Work out the finished part from the listing and answer in its coordinate system (mm). Give positions to 0.01 mm unless a question says otherwise; leave off trailing zeros. Loops run counter-clockwise (first coordinate to the right, second up) from the corner with the lowest first, then second, coordinate; pieces in that order, holes last. Notation, with made-up numbers: M -33.75,53.25 L 25.25,53.25 A19 ccw 25.25,80.25 Z; hole C -16.75,-24.5 d6. An arc over 180 degrees is marked long. Answer as a JSON object with one key per item and string values. Group by question number.
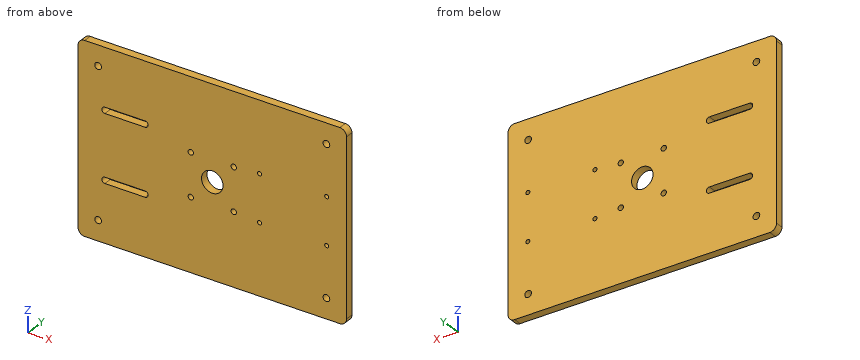
```python
from build123d import *

# Parameters (mm, degrees)
SKETCH2_W           = 200
SKETCH2_H           = 140
BOSS_EXTRUDE1_DEPTH = 6
FILLET1_R           = 5
SKETCH3_R           = 2.5
CUT_EXTRUDE1_DEPTH  = 123.21292894
SKETCH4_R           = 8
CUT_EXTRUDE2_DEPTH  = 123.21292894
SKETCH5_R           = 2
CUT_EXTRUDE3_DEPTH  = 123.21292894
CUT_EXTRUDE4_DEPTH  = 123.21292894
SKETCH7_R           = 1.5
CUT_EXTRUDE5_DEPTH  = 123.21292894


with BuildPart() as part:
    # Sketch2 → Boss-Extrude1 (new body)
    with BuildSketch(Plane(origin=(0, 0, 0), x_dir=(1, 0, 0), z_dir=(0, 1, 0))):
        Rectangle(SKETCH2_W, SKETCH2_H)
    extrude(amount=BOSS_EXTRUDE1_DEPTH)

    # Fillet1
    fillet1_edges = [part.edges().sort_by_distance(p)[0] for p in [
        (100, 3, 70),
        (-100, 3, 70),
        (-100, 3, -70),
        (100, 3, -70),
    ]]
    fillet(fillet1_edges, radius=FILLET1_R)

    # Sketch3 → Cut-Extrude1 (cut, through all)
    with BuildSketch(Plane(origin=(0, 6, 0), x_dir=(1, 0, 0), z_dir=(0, 1, 0))):
        with Locations(Location((-85, 55, 0), (0, 0, 270))):
            Circle(SKETCH3_R)
        with Locations(Location((-85, -55, 0), (0, 0, 90))):
            Circle(SKETCH3_R)
        with Locations(Location((85, -55, 0), (0, 0, 270))):
            Circle(SKETCH3_R)
        with Locations(Location((85, 55, 0), (0, 0, 90))):
            Circle(SKETCH3_R)
    extrude(amount=-CUT_EXTRUDE1_DEPTH, mode=Mode.SUBTRACT)

    # Sketch4 → Cut-Extrude2 (cut, through all)
    with BuildSketch(Plane(origin=(0, 6, 0), x_dir=(1, 0, 0), z_dir=(0, 1, 0))):
        with Locations(Location((0, 0, 0), (0, 0, 270))):
            Circle(SKETCH4_R)
    extrude(amount=-CUT_EXTRUDE2_DEPTH, mode=Mode.SUBTRACT)

    # Sketch5 → Cut-Extrude3 (cut, through all)
    with BuildSketch(Plane(origin=(0, 6, 0), x_dir=(1, 0, 0), z_dir=(0, 1, 0))):
        with Locations(Location((16, 16, 0), (0, 0, 270))):
            Circle(SKETCH5_R)
        with Locations(Location((16, -16, 0), (0, 0, 270))):
            Circle(SKETCH5_R)
        with Locations(Location((-16, -16, 0), (0, 0, 270))):
            Circle(SKETCH5_R)
        with Locations(Location((-16, 16, 0), (0, 0, 270))):
            Circle(SKETCH5_R)
    extrude(amount=-CUT_EXTRUDE3_DEPTH, mode=Mode.SUBTRACT)

    # Sketch6 → Cut-Extrude4 (cut, through all)
    with BuildSketch(Plane(origin=(0, 6, 0), x_dir=(1, 0, 0), z_dir=(0, 1, 0))):
        with BuildLine():
            Line((-80, 27.25), (-50, 27.25))
            ThreePointArc((-50, 27.25), (-47.75, 25), (-50, 22.75))
            Line((-50, 22.75), (-80, 22.75))
            ThreePointArc((-80, 22.75), (-82.25, 25), (-80, 27.25))
        make_face()
        with BuildLine():
            Line((-80, -22.75), (-50, -22.75))
            ThreePointArc((-50, -22.75), (-47.75, -25), (-50, -27.25))
            Line((-50, -27.25), (-80, -27.25))
            ThreePointArc((-80, -27.25), (-82.25, -25), (-80, -22.75))
        make_face()
    extrude(amount=-CUT_EXTRUDE4_DEPTH, mode=Mode.SUBTRACT)

    # Sketch7 → Cut-Extrude5 (cut, through all)
    with BuildSketch(Plane(origin=(0, 6, 0), x_dir=(1, 0, 0), z_dir=(0, 1, 0))):
        with Locations(Location((35.22226737, -17.5, 0), (0, 0, 270))):
            Circle(SKETCH7_R)
        with Locations(Location((35.22226737, 17.5, 0), (0, 0, 270))):
            Circle(SKETCH7_R)
        with Locations(Location((85.22226737, 17.5, 0), (0, 0, 270))):
            Circle(SKETCH7_R)
        with Locations(Location((85.22226737, -17.5, 0), (0, 0, 270))):
            Circle(SKETCH7_R)
    extrude(amount=-CUT_EXTRUDE5_DEPTH, mode=Mode.SUBTRACT)


solid = part.part
```
Item 1: A cutting plane is placed at D-D (y = 2.75). Give the number of separate pieces and of enclosed holes in the cut face, and give its area (3 significant figures).
Item 2: A cutting plane is placed at A-A (x = 16). Determine the outline of the cut face in (y, z), and give its area (3 significant figures).
Item 3: Given pin 1 Ø13 at (x, z) = (0, 0) entering from +Y, flat-ended and moving along its own axis, determine where the tip first touches the part or whether it passes through.
Item 4: A cutting plane is placed at B-B (z = 0). Determine the outline of the cut face in (x, y), and give its area (3 significant figures).
Item 5: Find the intervals of material crossed by probe 1 along X at (y, z) = (4.7, -55); probe 2 along Z at (x, y) = (-60, 0.5); probe 3 along Z at (x, y) = (-86, 4.85), in increasing order. Write a range as [from, to].
Item 6: A cutting plane is placed at C-C (x = -70.5). Determine the outline of the cut face in (y, z), and give its area (3 significant figures).
The answers:
{
 "1": {"separate pieces": "1", "enclosed holes": "15", "area": "27,300 mm^2"},
 "2": {"outline": "M 0,-70 L 6,-70 L 6,-18 L 0,-18 Z; M 0,-14 L 6,-14 L 6,14 L 0,14 Z; M 0,18 L 6,18 L 6,70 L 0,70 Z", "area": "792 mm^2"},
 "3": {"pin 1": "passes through"},
 "4": {"outline": "M -100,0 L -8,0 L -8,6 L -100,6 Z; M 8,0 L 100,0 L 100,6 L 8,6 Z", "area": "1,100 mm^2"},
 "5": {"probe 1": "x = [-100, -87.5], [-82.5, 82.5], [87.5, 100]", "probe 2": "z = [-70, -27.25], [-22.75, 22.75], [27.25, 70]", "probe 3": "z = [-70, -57.29], [-52.71, 52.71], [57.29, 70]"},
 "6": {"outline": "M 0,-70 L 6,-70 L 6,-27.25 L 0,-27.25 Z; M 0,-22.75 L 6,-22.75 L 6,22.75 L 0,22.75 Z; M 0,27.25 L 6,27.25 L 6,70 L 0,70 Z", "area": "786 mm^2"}
}
